```python
from build123d import *

# Parameters (mm, degrees)
F0_R     = 254
F1_DEPTH = 254


with BuildPart() as f1:
    # F0 (on Front) → F1 (new body)
    with BuildSketch(Plane.XZ):
        with BuildLine():
            ThreePointArc((0, 127), (37.197439, 37.197439), (127, 0))
            Line((127, 0), (1651, 0))
            ThreePointArc((1651, 0), (1740.802561, 37.197439), (1778, 127))
            Line((1778, 127), (1778, 381))
            Line((1778, 381), (2047.407684, 650.407684))
            Line((2047.407684, 650.407684), (1778, 919.815367))
            Line((1778, 919.815367), (1508.592316, 650.407684))
            Line((1508.592316, 650.407684), (1328.987194, 830.012806))
            Line((1328.987194, 830.012806), (1598.394878, 1099.42049))
            Line((1598.394878, 1099.42049), (1388.600741, 1309.214626))
            Line((1388.600741, 1309.214626), (1143, 1016))
            Line((1143, 1016), (889, 1016))
            Line((889, 1016), (889, 762))
            Line((889, 762), (762, 762))
            Line((762, 762), (762, 1016))
            Line((762, 1016), (381, 1016))
            ThreePointArc((381, 1016), (291.197439, 978.802561), (254, 889))
            Line((254, 889), (254, 508))
            Line((254, 508), (127, 508))
            ThreePointArc((127, 508), (37.197439, 470.802561), (0, 381))
            Line((0, 381), (0, 127))
        make_face()
        with Locations((825.5, 381)):
            Circle(F0_R, mode=Mode.SUBTRACT)
    extrude(amount=F1_DEPTH)


solid = f1.part
```
CAD build for the part. Positions are in the model's coordinates, mm. A direction names the side the tool comes from. Coordinates: 2 decimals unless noted, no trailing zeros. Loops run counter-clockwise (first coordinate to the right, second up) from the corner with the lowest first, then second, coordinate; pieces in that order, holes last. Notation, with made-up numbers: (-23.5, 52) - (34.5, 52) arc R31 ccw to (34.5, 78) - close; hole circle Ø7 at (74, -35.75). An arc over 180 degrees is marked (long way). Use CSV: the item, a comma, the result in double quotes. Start each with the question number.
Q1. Cut at D-D, the plane z = 854.5. List the corners of the cut face in (x, y).
Q2. 3-axis set-ups, long thin cutter, end or side, ignore diameter. For faces 4 (the flat face through (826, -125, 762)), 5 (the flat face through (1778, -125, 252)), 6 (the flat face through (1420, -125, 739)): which of +Z, -Z, +X, -X, +Y, -Y reach the whole face in a straight line?
Q3. Two-plate mould, pull along X, no slides. Class faces 1 (the flat face through (254, -125, 701)), 2 (the flat face through (878, -125, 0)), 3 (the flat face through (889, -125, 891)): +X half, -X half, draft (parallel to the pull), parting line (faces both ways), or undercut.
Q4. Probe probe 1 along Z at (x, y) = (831.5, -186); probe 2 along Z at (x, y) = (825, -104); probe 3 along X at (y, z) = (-183.5, 813). List the from-to ranges inside material, lowest first. Write a range as from..to.
Q5. Cut at C-C, the plane z = 182. List the corners of the cut face in (x, y).
Q6. Cut at B-B, the plane y = -132.5. List the corners of the cut face in (x, z).
Q7. Cut at A-A, the plane x = 825.5. List the corners of the cut face in (y, z).
Q8. Drop a flat-ended pin along its axis: P1, Ø2, axis at y = -73.5, z = 779, coming from the -X side. Give the stop position or say it passes through.
Here are the results:
1,outline,"(254, -254) - (762, -254) - (762, 0) - (254, 0) - close; (889, -254) - (1353.47, -254) - (1353.47, 0) - (889, 0) - close; (1712.68, -254) - (1843.32, -254) - (1843.32, 0) - (1712.68, 0) - close"
2,face 4,"+Z, +Y, -Y"
2,face 5,"-Z, +X, +Y, -Y"
2,face 6,"+Y, -Y"
3,face 1,"-X half"
3,face 2,"draft"
3,face 3,"undercut"
4,probe 1,"0..127.07, 634.93..762"
4,probe 2,"0..127, 635..762"
4,probe 3,"254..762, 889..1346, 1671.18..1884.82"
5,outline,"(0, -254) - (667.66, -254) - (667.66, 0) - (0, 0) - close; (983.34, -254) - (1778, -254) - (1778, 0) - (983.34, 0) - close"
6,outline,"(0, 127) arc R127 ccw to (127, 0) - (1651, 0) arc R127 ccw to (1778, 127) - (1778, 381) - (2047.41, 650.41) - (1778, 919.82) - (1508.59, 650.41) - (1328.99, 830.01) - (1598.39, 1099.42) - (1388.6, 1309.21) - (1143, 1016) - (889, 1016) - (889, 762) - (762, 762) - (762, 1016) - (381, 1016) arc R127 ccw to (254, 889) - (254, 508) - (127, 508) arc R127 ccw to (0, 381) - close; hole circle Ø508 at (825.5, 381)"
7,outline,"(-254, 0) - (0, 0) - (0, 127) - (-254, 127) - close; (-254, 635) - (0, 635) - (0, 762) - (-254, 762) - close"
8,P1,"x = 254"
